The drawing under review shows one solid part. Ordinate dimensions are in mm from its lowest x, y, z. A direction names the side the tool comes from. Give positions to 0.01 mm unless a question says otherwise; leave off trailing zeros. Order: outer loops, then holes, each group sorted by start corner. A loop starts at its lowest first (then second) coordinate and runs counter-clockwise, first axis right, second up. Notation, with made-up numbers: (87, -18.5) - (130, -18.5) arc R15 ccw to (130, 5.5) - close; hole circle Ø4 at (18.5, 57). An arc over 180 degrees is marked (long way). Use CSV: the item, a comma, the result in double quotes. Start each with the question number.
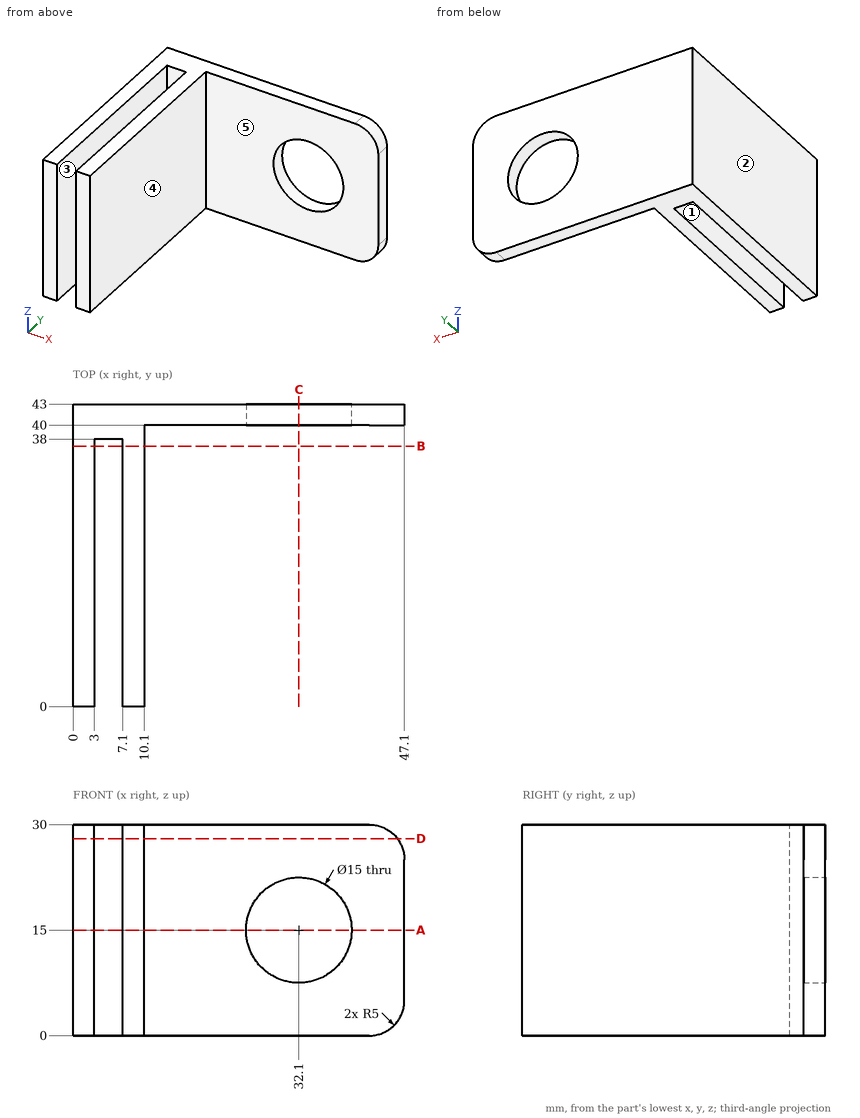
1. Mouldability with a two-part tool opening along X and no side actions: class the marked faces 3, 4 and 5 as pulls with the +X half, pulls with the -X half, needs draft (parallel to the pull), parting line crosses it, or undercut.
2. Consider section D-D (z = 28). Give the boundary of the cut face in (x, y), and give its area (4 significant figures).
3. Clearance check with flat-ended pins moving along their axes: pin 1 (4 mm diameter, centred on y = 7.5, z = 13.5, fed in from +X); pin 2 (10 mm diameter, centred on x = 39, y = 30.5, fed in from +Z); pin 3 (8 mm diameter, centred on x = 34, z = 3.5, fed in from -Y); pin 4 (2 mm diameter, centred on x = 38, z = 11, fed in from +Y). State where each tip first meets the part, or that it passes through.
4. Consider section C-C (x = 32.1). Give the boundary of the cut face in (y, z).
5. Consider section B-B (y = 37). Give the boundary of the cut face in (x, z), and give its area (3 significant figures).
6. Consider section A-A (z = 15). Give the boundary of the cut face in (x, y).
7. Tool access review of the marked faces 1 and 2: name each direction out of +Z, -Z, +X, -X, +Y, -Y from which nothing blocks a thin tool from reaching the whole face with its end or side.
8. To check wall thickness, follow L1, parallel to X at y = 28, z = 17.5; L2, parallel to Z at x = 32, y = 41; L3, parallel to Y at x = 12, z = 24. State the ranges of each line that lie inside material, in increasing order. Write a range as [from, to].
Answers follow:
1,face 3,"undercut"
1,face 4,"pulls with the +X half"
1,face 5,"needs draft"
2,outline,"(0, 0) - (3, 0) - (3, 38) - (7.1, 38) - (7.1, 0) - (10.1, 0) - (10.1, 40) - (46.1, 40) - (46.1, 43) - (0, 43) - close"
2,area,"386.5 mm^2"
3,pin 1,"stops at x = 10.1"
3,pin 2,"passes through"
3,pin 3,"stops at y = 40"
3,pin 4,"stops at y = 43"
4,outline,"(40, 0) - (43, 0) - (43, 7.5) - (40, 7.5) - close; (40, 22.5) - (43, 22.5) - (43, 30) - (40, 30) - close"
5,outline,"(0, 0) - (3, 0) - (3, 30) - (0, 30) - close; (7.1, 0) - (10.1, 0) - (10.1, 30) - (7.1, 30) - close"
5,area,"180 mm^2"
6,outline,"(0, 0) - (3, 0) - (3, 38) - (7.1, 38) - (7.1, 0) - (10.1, 0) - (10.1, 40) - (24.6, 40) - (24.6, 43) - (0, 43) - close; (39.6, 40) - (47.1, 40) - (47.1, 43) - (39.6, 43) - close"
7,face 1,"+Z, -Z, -Y"
7,face 2,"+Z, -Z, -X, +Y, -Y"
8,L1,"x = [0, 3], [7.1, 10.1]"
8,L2,"z = [0, 7.5], [22.5, 30]"
8,L3,"y = [40, 43]"
